```python
from build123d import *

# Parameters (mm, degrees)
F0_W   = 23
F0_H   = 3
F0_W_2 = 6
F0_W_3 = 13


# Not quite as in the source:
# - a feature names something its author has since deleted; it is built from what else it names


with BuildPart() as f1:
    # F0 (on Front) → F1 (revolve)
    with BuildSketch(Plane.XZ):
        Polygon((25, 5), (0, 5), (0, 3), (0, 0), (25, 0), (25, 3), align=None)
        with Locations((-11.5, 1.5)):
            Rectangle(F0_W, F0_H)
        with Locations((-26, 1.5)):
            Rectangle(F0_W_2, F0_H)
        with Locations((31.5, 1.5)):
            Rectangle(F0_W_3, F0_H)
    revolve(axis=Axis((1, 0, 0), (1, 0, 0)))


solid = f1.part
```
Verification items for the finished model (mm, model axes). A direction names the side the tool comes from. Round coordinates to 2 decimals unless told otherwise and drop trailing zeros. Write each loop counter-clockwise with the first axis right and the second up, starting at its lowest first coordinate (ties: lowest second). Pieces come first, ordered by that corner, then holes. Notation, with made-up numbers: (-28, -8) -> (-9, -8) arc R21 cw to (-9, -2) -> close; hole circle Ø1 at (37.5, 51). An arc over 180 degrees is marked (long way). Write each question's results on one line, items separated by ' | '. Start each with the question number.
1. Set-up check for faces 1 (the cylindrical face through (-15, 0, -3)), 2 (the flat face through (25, -0.1, -3.3)), 3 (the flat face through (-29, 0, 0)): record each of +Z, -Z, +X, -X, +Y, -Y from which the full face is reachable in a straight line by a thin tool's end or side.
2. Cross-section at D-D (z = -4). Enter the section's corners in (x, y), then the cut area to 3 significant figures.
3. Material ranges on probe 1 along X at (y, z) = (-2, 4.25); probe 2 along Z at (x, y) = (-2.5, 0), recorded low to high. Write a range as from..to.
4. Cross-section at C-C (x = -9). Enter the section's corners in (y, z), then the cut area to 3 significant figures.
5. Depth check by flat-ended pin: P1, Ø1, axis at x = -22, z = -1, coming from the +Y side; P2, Ø2, axis at x = -20, y = 2, coming from the -Z side; P3, Ø2, axis at x = 30, z = -2.5, coming from the -Y side. Enter the tip coordinate at first touch or a pass-through.
6. Cross-section at A-A (z = 0). Enter the section's corners in (x, y).
Solutions:
1) face 1: -X | face 2: +X | face 3: +Z, -Z, -X, +Y, -Y
2) outline: (0, -3) -> (25, -3) -> (25, 3) -> (0, 3) -> close | area: 150 mm2
3) probe 1: x = 0..25 | probe 2: z = -3..3
4) outline: circle Ø6 at (0, 0) | area: 28.3 mm2
5) P1: stops at y = 2.96 | P2: stops at z = -2.83 | P3: stops at y = -2.6
6) outline: (-29, -3) -> (0, -3) -> (0, -5) -> (25, -5) -> (25, -3) -> (38, -3) -> (38, 3) -> (25, 3) -> (25, 5) -> (0, 5) -> (0, 3) -> (-29, 3) -> close
